```python
from build123d import *

# Parameters (mm, degrees)
SKETCH1_W           = 76.879071809
SKETCH1_H           = 97.396637597
BOSS_EXTRUDE1_DEPTH = 20
SKETCH2_R           = 7.5
CUT_EXTRUDE1_DEPTH  = 20
FILLET2_R           = 5
FILLET3_R           = 5
FILLET4_R           = 5
FILLET5_R           = 5
SKETCH3_R           = 2.996522069
BOSS_EXTRUDE2_DEPTH = 5
FILLET7_R           = 2.5


with BuildPart() as part:
    # Sketch1 → Boss-Extrude1 (new body)
    with BuildSketch(Plane.XY):
        with Locations((36.214739615, -28.675152186)):
            Rectangle(SKETCH1_W, SKETCH1_H)
    extrude(amount=BOSS_EXTRUDE1_DEPTH)

    # Sketch2 → Cut-Extrude1 (cut)
    with BuildSketch(Plane.XY.offset(20)):
        with Locations((36.214739614, -28.675152186)):
            Circle(SKETCH2_R)
    extrude(amount=-CUT_EXTRUDE1_DEPTH, mode=Mode.SUBTRACT)

    # Fillet2
    fillet2_edges = [part.edges().sort_by_distance(p)[0] for p in [
        (74.654275519, 20.023166613, 10),
    ]]
    fillet(fillet2_edges, radius=FILLET2_R)

    # Fillet3
    fillet3_edges = [part.edges().sort_by_distance(p)[0] for p in [
        (74.654275519, -31.175152186, 20),
        (33.714739614, 20.023166613, 20),
        (73.189809425, 18.558700519, 20),
    ]]
    fillet(fillet3_edges, radius=FILLET3_R)

    # Fillet4
    fillet4_edges = [part.edges().sort_by_distance(p)[0] for p in [
        (33.714739614, 20.023166613, 0),
        (73.189809425, 18.558700519, 0),
        (74.654275519, -31.175152186, 0),
    ]]
    fillet(fillet4_edges, radius=FILLET4_R)

    # Fillet5
    fillet5_edges = [part.edges().sort_by_distance(p)[0] for p in [
        (-2.22479629, -31.175152186, 20),
        (-2.22479629, 20.023166613, 10),
        (-2.22479629, 18.558700519, 18.535533906),
        (-2.22479629, -31.175152186, 0),
        (-2.22479629, 18.558700519, 1.464466094),
    ]]
    fillet(fillet5_edges, radius=FILLET5_R)

    # Sketch3 → Boss-Extrude2 (add)
    with BuildSketch(Plane(origin=(0, 20.023166613, 0), x_dir=(1, 0, 0), z_dir=(0, 1, 0))):
        with Locations(Location((6.286432744, -10, 0), (0, 0, 90))):
            Circle(SKETCH3_R)
    extrude(amount=BOSS_EXTRUDE2_DEPTH)

    # Fillet7
    fillet7_edges = [part.edges().sort_by_distance(p)[0] for p in [
        (6.286432744, 25.023166613, 12.996522069),
    ]]
    fillet(fillet7_edges, radius=FILLET7_R)


solid = part.part
```
CAD build for the part. Positions are in the model's coordinates, mm. A direction names the side the tool comes from. Round coordinates to 2 decimals unless told otherwise and drop trailing zeros. Loops run counter-clockwise (first coordinate to the right, second up) from the corner with the lowest first, then second, coordinate; pieces in that order, holes last. Notation, with made-up numbers: M -16,52.25 L 2,52.25 A18 ccw 2,57.25 Z; hole C 44.5,31.5 d4. An arc over 180 degrees is marked long. Return JSON: item names as keys, results as strings. Group by question number.
(1) Drop a flat-ended pin along its axis: P1, Ø3, axis at x = 20, z = 8, coming from the +Y side. Give the stop position or say it passes through.
(2) Saw through at A-A, the plane y = -31.5. List the corners of the cut face in (x, z).
(3) Saw through at D-D, the plane z = 2.5. List the corners of the cut face in (x, y), and give its area (3 significant figures).
(4) Tool access for faces 1 (the cylindrical face through (-0.799, -31.822, 1.504)), 2 (the cylindrical face through (7.43, 21.26, 7.23)): list every direction of +Z, -Z, +X, -X, +Y, -Y with a clear straight run to the whole face (end or side of a thin tool).
(5) Saw through at C-C, the plane z = 17.75. List the corners of the cut face in (x, y).
(6) Mould opens along Y. For faces 3 (the cylindrical face through (30.263, -33.239, 10.14)), 4 (the flat face through (74.654, -32, 10)), 5 (the flat face through (36, -77.373, 10)) say: +Y half, -Y half, draft (parallel to the pull), parting line (faces both ways), or undercut.
(7) Wall check: probe 1 along Y at (x, z) = (36, 4.75); probe 2 along Y at (x, z) = (26.5, 9.75); probe 3 along X at (y, z) = (-59, 4.5). Give the ranges that are in metal, low to high. Write a range as [from, to].
(8) Saw through at B-B, the plane x = 23. List the corners of the cut face in (y, z).
Answer list:
{
 "1": {"P1": "y = 20.02"},
 "2": {"outline": "M -2.22,5 A5 ccw 2.78,0 L 29.27,0 L 29.27,20 L 2.78,20 A5 ccw -2.22,15 Z; M 43.16,0 L 69.65,0 A5 ccw 74.65,5 L 74.65,15 A5 ccw 69.65,20 L 43.16,20 Z"},
 "3": {"outline": "M -1.55,-77.37 L 73.98,-77.37 L 73.98,15.02 A4.33 ccw 69.65,19.35 L 2.78,19.35 A4.33 ccw -1.55,15.02 Z; hole C 36.21,-28.68 d15", "area": "7,120 mm2"},
 "4": {"face 1": "-Z, -X, +Y, -Y", "face 2": "+Y"},
 "5": {"outline": "M -1.4,-77.37 L 73.83,-77.37 L 73.83,15.02 A4.18 ccw 69.65,19.2 L 2.78,19.2 A4.18 ccw -1.4,15.02 Z; hole C 36.21,-28.68 d15"},
 "6": {"face 3": "undercut", "face 4": "draft", "face 5": "-Y half"},
 "7": {"probe 1": "[-77.37, -36.17], [-21.18, 20.02]", "probe 2": "[-77.37, 20.02]", "probe 3": "[-2.2, 74.63]"},
 "8": {"outline": "M -77.37,0 L 15.02,0 A5 ccw 20.02,5 L 20.02,15 A5 ccw 15.02,20 L -77.37,20 Z"}
}
